Autodesk Inventor part; units mm, degrees
ref_plane "YZ Plane" through (0, 0, 0) normal (1, 0, 0) x (0, 1, 0)
ref_plane "XZ Plane" through (0, 0, 0) normal (0, 1, 0) x (-1, 0, 0)
ref_plane "XY Plane" through (0, 0, 0) normal (0, 0, 1) x (1, 0, 0)
sketch "Sketch1" plane through (0, 0, 0) normal (0, 0, 1) x (1, 0, 0)
  circle A0 centre (0, 0) radius 5
  dimension "d0" = 10
extrude "Extrusion1" add sketch "Sketch1" along normal blind 2
sketch "Sketch2" plane through (0, 0, 2) normal (0, 0, 1) x (1, 0, 0)
  circle A0 centre (0, 0) radius 5
  circle A1 centre (0, 0) radius 3.9
  dimension "d4" = 7.8
extrude "Extrusion2" add sketch "Sketch2" along normal blind 7 contours A1
sketch "Sketch3" plane through (0, 0, 9) normal (0, 0, 1) x (1, 0, 0)
  circle A0 centre (0, 0) radius 3.9
  circle A1 centre (0, 0) radius 1.55
  dimension "d9" = 3.1
extrude "Extrusion3" cut sketch "Sketch3" against normal through all contours A1
properties part number "z idler insert"
Can you work these out from the model? Positions are in its coordinate system, mm. Give positions to 0.01 mm unless a question says otherwise; leave off trailing zeros. Order: outer loops, then holes, each group sorted by start corner. A loop starts at its lowest first (then second) coordinate and runs counter-clockwise, first axis right, second up. Notation, with made-up numbers: M -10,-12 L 31,-12 A31 ccw 31,18 Z; hole C 79.25,48.25 d4. An arc over 180 degrees is marked long. Write item = value, one per line. Start each with the question number.
Q1. Suppose I cut it at A-A (x = 0). Write out the boundary of the cut face in (y, z).
Q2. Suppose I cut it at D-D (y = -2.25). Write out the boundary of the cut face in (x, z).
Q3. Suppose I cut it at C-C (z = 1.5). Write out the boundary of the cut face in (x, y).
Q4. I need wall thicknesses on probe 1 along Y at (x, z) = (0, 4); probe 2 along Y at (x, z) = (0, 1.75); probe 3 along Z at (x, y) = (0.75, -4.25). Which ranges of each line are inside material? Lowest first, please. Write a range as [from, to].
Q5. We'd pull the mould along Y, two halves only. Please class faces 1 (the cylindrical face through (-2.87, -2.64, 5.45)), 2 (the flat face through (3, -3, 2)), 3 (the cylindrical face through (0.715, -1.375, 4.563)): pulls with the +Y half, pulls with the -Y half, needs draft (parallel to the pull), parting line crosses it, or undercut.
Q6. Will these pins go through, and if not, where does the flat tip stop? pin 1 Ø2 at (x, y) = (2.5, 2.5) entering from -Z; pin 2 Ø2 at (x, z) = (3, 5) entering from -Y; pin 3 Ø4 at (y, z) = (0, 8) entering from -X.
Check result:
q1.outline = M -5,0 L -1.55,0 L -1.55,9 L -3.9,9 L -3.9,2 L -5,2 Z; M 1.55,0 L 5,0 L 5,2 L 3.9,2 L 3.9,9 L 1.55,9 Z
q2.outline = M -4.47,0 L 4.47,0 L 4.47,2 L 3.19,2 L 3.19,9 L -3.19,9 L -3.19,2 L -4.47,2 Z
q3.outline = C 0,0 d10; hole C 0,0 d3.1
q4.probe_1 = [-3.9, -1.55], [1.55, 3.9]
q4.probe_2 = [-5, -1.55], [1.55, 5]
q4.probe_3 = [0, 2]
q5.face_1 = parting line crosses it
q5.face_2 = needs draft
q5.face_3 = undercut
q6.pin_1 = 0
q6.pin_2 = -3.35
q6.pin_3 = -3.9
